```python
from build123d import *


with BuildPart() as part:
    # 草图1 → 旋转1 (revolve)
    with BuildSketch(Plane(origin=(0, 0, 0), x_dir=(1, 0, 0), z_dir=(0, 1, 0)), mode=Mode.PRIVATE) as revolve_1_sk:
        with BuildLine():
            Line((0, 25), (0, 10))
            Line((0, 10), (2, 10))
            Line((2, 10), (2, 0))
            Line((2, 0), (25, 0))
            Line((25, 0), (25, 3))
            Line((25, 3), (13, 3))
            Line((13, 3), (13, 6))
            Line((13, 6), (12, 6))
            Line((12, 6), (12, 25))
            ThreePointArc((12, 25), (6, 27.708497378), (0, 25))
        make_face()
    revolve(revolve_1_sk.sketch.rotate(Axis((0, 0, 0), (1, 0, 0)), 180), axis=Axis((0, 0, 0), (1, 0, 0)))


solid = part.part
```
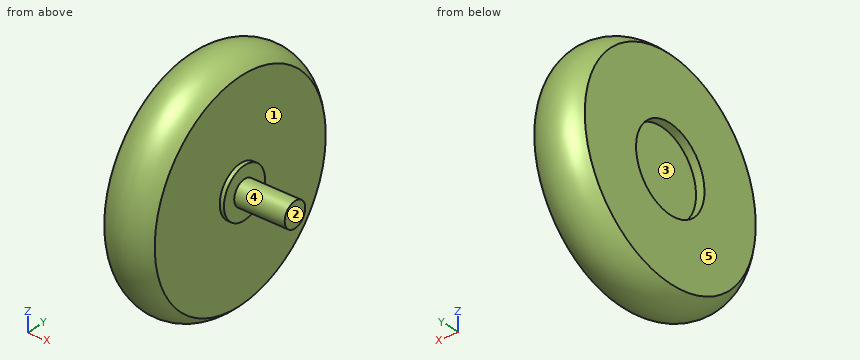
Model file for the job. Use its own axes, mm. Face numbers are marked on the shaded views. A direction names the side the tool comes from. Give positions to 0.01 mm unless a question says otherwise; leave off trailing zeros. Loops run counter-clockwise (first coordinate to the right, second up) from the corner with the lowest first, then second, coordinate; pieces in that order, holes last. Notation, with made-up numbers: M 62.5,48 L 84.5,48 A6 cw 84.5,59 Z; hole C 23.5,55.5 d10. An arc over 180 degrees is marked long. Use one line per item in the form item = value.
Item 1: Slice it at A-A on z = 0. List the corners of the cut face in (x, y), and give its area (3 significant figures).
Filled in:
outline = M 0,-25 A8 ccw 12,-25 L 12,-6 L 13,-6 L 13,-3 L 25,-3 L 25,3 L 13,3 L 13,6 L 12,6 L 12,25 A8 ccw 0,25 L 0,10 L 2,10 L 2,-10 L 0,-10 Z
area = 689 mm^2
Item 2: Which spindle directions (+Z, -Z, +X, -X, +Y, -Y) get a long thin tool onto all of the face, cutting with end or side? Do the marked faces 1 and 2. Say none if no direction does.
Filled in:
face_1 = +X
face_2 = +Z, -Z, +X, +Y, -Y
Item 3: Slice it at C-C on x = 5.5. List the corners of the cut face in (y, z), and give its area (3 significant figures).
Filled in:
outline = C 0,0 d55.39
area = 2,410 mm^2
Item 4: Two-plate mould, pull along Z, no slides. Class the marked faces 3, 4 and 5: released by +Z, released by -Z, zero draft, split by the parting line, or undercut.
Filled in:
face_3 = undercut
face_4 = split by the parting line
face_5 = zero draft
Item 5: Flat gauge pins, fed straight in: pin 1 Ø6 at (y, z) = (-7, 19) entering from +X; pin 2 Ø8 at (x, z) = (15.5, 17.5) entering from +Y; pin 3 Ø6 at (x, z) = (11.5, 16) entering from -Y. Where does each tip first touch, or does it go through?
Filled in:
pin_1 = 12
pin_2 = 19.56
pin_3 = -23.12
Item 6: Drill centre lines: L1, parallel to X at y = 5.5, z = -23; L2, parallel to X at y = -1, z = 3; L3, parallel to Y at x = 0.95, z = 0. Where is each one in solid material? Low to high.
Filled in:
L1 = 0 to 12
L2 = 2 to 13
L3 = -25.91 to -10, 10 to 25.91
